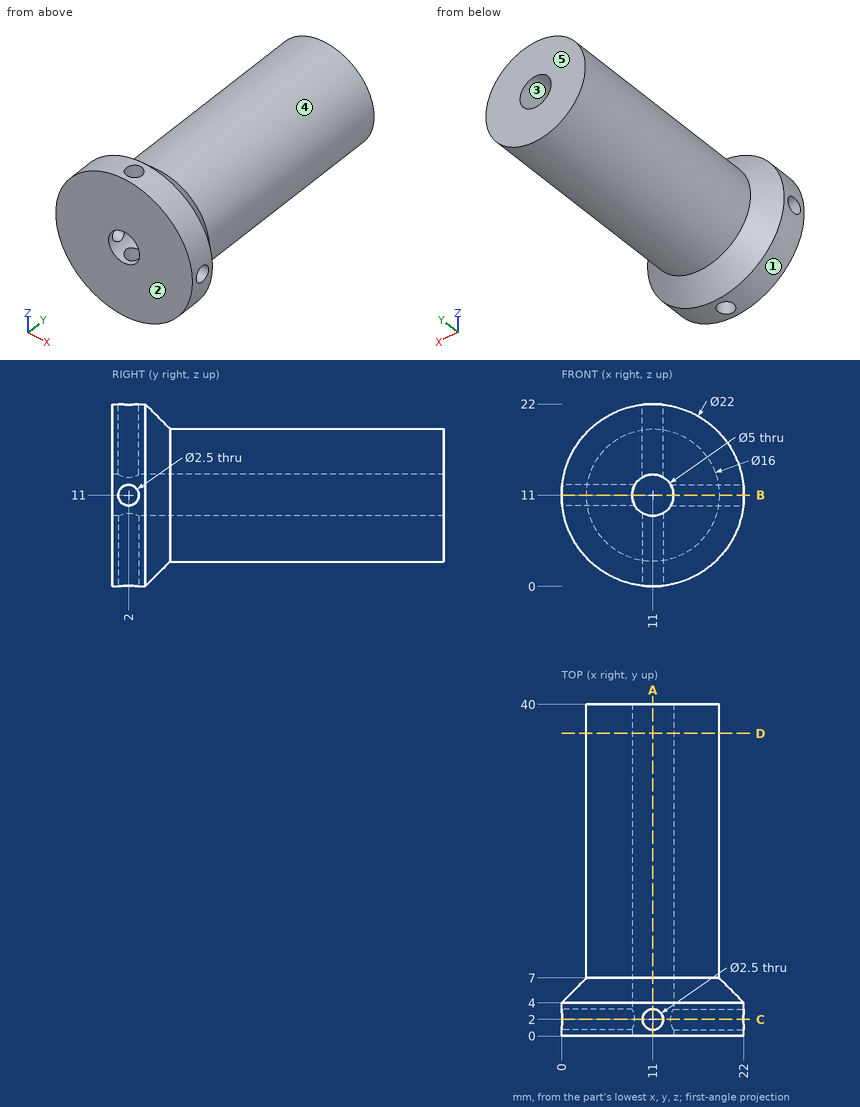
Print and shaded views of the part. All mm, measured from the part's lowest x, y and z. A direction names the side the tool comes from. Round coordinates to 2 decimals unless told otherwise and drop trailing zeros. Loops run counter-clockwise (first coordinate to the right, second up) from the corner with the lowest first, then second, coordinate; pieces in that order, holes last. Notation, with made-up numbers: M -15.5,-1 L 20.5,-1 A26 cw 20.5,37 Z; hole C 5.25,-18.5 d7. An arc over 180 degrees is marked long. One line per question, with ' | ' between items.
1) Band-saw the part on D-D (y = 36.5). Give the cut face in (x, z), then the cut area to 3 significant figures.
Solved:
outline: C 11,11 d16; hole C 11,11 d5 | area: 181 mm²
2) Mould opens along Z. For the marked faces 1, 2 and 3 say: +Z half, -Z half, draft (parallel to the pull), parting line (faces both ways), or undercut.
Solved:
face 1: parting line | face 2: draft | face 3: undercut
3) Band-saw the part on C-C (y = 2). Give the cut face in (x, z).
Solved:
outline: M 0.07,9.75 A11 ccw 9.75,0.07 L 9.75,8.83 A2.5 cw 8.83,9.75 Z; M 0.07,12.25 L 8.83,12.25 A2.5 cw 9.75,13.17 L 9.75,21.93 A11 ccw Z; M 12.25,0.07 A11 ccw 21.93,9.75 L 13.17,9.75 A2.5 cw 12.25,8.83 Z; M 12.25,13.17 A2.5 cw 13.17,12.25 L 21.93,12.25 A11 ccw 12.25,21.93 Z
4) Band-saw the part on B-B (z = 11). Give the cut face in (x, y), then the cut area to 4 significant figures.
Solved:
outline: M 0,0 L 8.5,0 L 8.5,0.75 L 0,0.75 Z; M 0,3.25 L 8.5,3.25 L 8.5,40 L 3,40 L 3,7 L 0,4 Z; M 13.5,0 L 22,0 L 22,0.75 L 13.5,0.75 Z; M 13.5,3.25 L 22,3.25 L 22,4 L 19,7 L 19,40 L 13.5,40 Z | area: 430.5 mm²
5) Band-saw the part on A-A (x = 11). Give the cut face in (y, z).
Solved:
outline: M 0,0 L 0.75,0 L 0.75,8.5 L 0,8.5 Z; M 0,13.5 L 0.75,13.5 L 0.75,22 L 0,22 Z; M 3.25,0 L 4,0 L 7,3 L 40,3 L 40,8.5 L 3.25,8.5 Z; M 3.25,13.5 L 40,13.5 L 40,19 L 7,19 L 4,22 L 3.25,22 Z
6) Flat gauge pins, fed straight in: pin 1 (3 mm diameter, centred on x = 11, y = 2, fed in from +Z); pin 2 (1.5 mm diameter, centred on x = 11, y = 19, fed in from +Z); pin 3 (2 mm diameter, centred on y = 2, z = 11, fed in from +X); pin 4 (10 mm diameter, centred on x = 18.5, y = 22.5, fed in from -Z). Where does each tip first touch, or does it go through?
Solved:
pin 1: stops at z = 22 | pin 2: stops at z = 19 | pin 3: passes through | pin 4: stops at z = 3.4
7) 3-axis set-ups, long thin cutter, end or side, ignore diameter. For the marked faces 4 and 5: which of +Z, -Z, +X, -X, +Y, -Y reach the whole face in a straight line?
Solved:
face 4: +Y | face 5: +Z, -Z, +X, -X, +Y
8) Drill centre lines: line 1 along Z through (x, y) = (11, 21); line 2 along Y through (x, z) = (11, 6); line 3 along Y through (x, z) = (14.25, 10). Where is each one in solid material? Low to high.
Solved:
line 1: z = 3 to 8.5, 13.5 to 19 | line 2: y = 0 to 0.75, 3.25 to 40 | line 3: y = 0 to 1.25, 2.75 to 40
